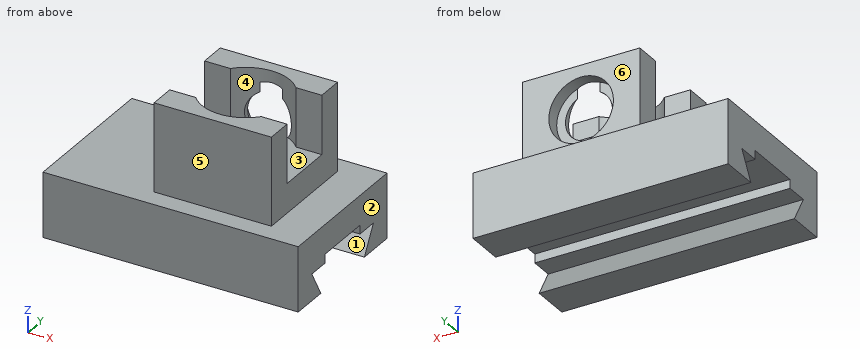
```python
from build123d import *

# Parameters (mm, degrees)
SKETCH1_W         = 87
SKETCH1_H         = 50.982
BASE_YELLOW_DEPTH = 22
SKETCH5_W         = 40
SKETCH5_H         = 38
BASE_RED_DEPTH    = 30
BASE_TURKIZ_DEPTH = 88
SKETCH2_R         = 11
COUNTERBOR_DEPTH  = 4.5
SKETCH7_R         = 15
SKETCH7_W         = 40
SKETCH7_H         = 20
BASE_PURPLE_DEPTH = 20
SKETCH2_5_R       = 8
COUNTERBOR2_DEPTH = 8


with BuildPart() as part:
    # Sketch1 → base-yellow (new body)
    with BuildSketch(Plane.XY):
        Rectangle(SKETCH1_W, SKETCH1_H)
    extrude(amount=-BASE_YELLOW_DEPTH)

    # Sketch5 → base-red (add)
    with BuildSketch(Plane.XY):
        with Locations((10.5, 0)):
            Rectangle(SKETCH5_W, SKETCH5_H)
    extrude(amount=BASE_RED_DEPTH)

    # Sketch8 → base-turkiz (cut, through all)
    with BuildSketch(Plane.ZY.offset(43.5)):
        Polygon((-10, 10), (-10, -10), (-13, -10), (-13, -17.696152423), (-22, -12.5), (-22, 12.5), (-13, 17.696152423), (-13, 10), align=None)
    extrude(amount=-BASE_TURKIZ_DEPTH, mode=Mode.SUBTRACT)

    # Sketch2 → counterbor (cut)
    with BuildSketch(Plane(origin=(0, 19, -19), x_dir=(1, 0, 0), z_dir=(0, -1, 0))):
        with Locations((10.5, 34)):
            Circle(SKETCH2_R)
    extrude(amount=COUNTERBOR_DEPTH, mode=Mode.SUBTRACT)

    # Sketch7 → base-purple (cut)
    with BuildSketch(Plane.XY.offset(30)):
        with Locations((10.5, 0)):
            Circle(SKETCH7_R)
        with Locations((10.5, 0)):
            Rectangle(SKETCH7_W, SKETCH7_H)
    extrude(amount=-BASE_PURPLE_DEPTH, mode=Mode.SUBTRACT)

    # Sketch2<5> → counterbor2 (cut)
    with BuildSketch(Plane(origin=(0, 19, -19), x_dir=(1, 0, 0), z_dir=(0, -1, 0))):
        with Locations((10.5, 34)):
            Circle(SKETCH2_5_R)
    extrude(amount=COUNTERBOR2_DEPTH, mode=Mode.SUBTRACT)


solid = part.part
```
Could you check a few things on this model? Use its own coordinates, in mm. Face numbers are marked on the shaded views. A direction names the side the tool comes from. Round coordinates to 2 decimals unless told otherwise and drop trailing zeros. Loops run counter-clockwise (first coordinate to the right, second up) from the corner with the lowest first, then second, coordinate; pieces in that order, holes last.
Q1. I want a section at A-A (x = 10.5). Write out the boundary of the cut face in (y, z), and give its area (3 significant figures).
Q2. I want a section at D-D (y = -8). Write out the boundary of the cut face in (x, z), and give its area (3 significant figures).
Q3. For P1, Ø2.5, axis at x = -4.5, z = 22.5, coming from the +Y side; P2, Ø4.5, axis at x = 26.5, z = 22, coming from the -Y side; P3, Ø6, axis at y = 10.5, z = 20.5, coming from the +X side, each with a flat end and sliding along its axis, tell me the tip position at first contact or that it passes through.
Q4. On a 3-axis mill with a long thin cutter (end or side, diameter ignored), from which of +Z, -Z, +X, -X, +Y, -Y can I reach the whole of each face in a straight line? I mean the marked faces 4, 5 and 6. Say none if no direction works.
Q5. I want a section at B-B (x = 27.5). Write out the boundary of the cut face in (y, z).
Q6. I want a section at C-C (z = 19.5). Write out the boundary of the cut face in (x, y).
Q7. Please list where these lines run through material, in increasing order: L1, parallel to X at y = 17.35, z = 15; L2, parallel to Z at x = 10.5, y = 15.55; L3, parallel to Z at x = 10.5, y = 15.7.
Q8. Thinking about a two-plate mould opening in Z: for the marked faces 1, 2 and 3, which applies, pulls with the +Z half, pulls with the -Z half, needs draft (parallel to the pull), parting line crosses it, or undercut?
Answer below:
1. outline: (-25.49, -22) - (-12.5, -22) - (-17.7, -13) - (-10, -13) - (-10, -10) - (10, -10) - (10, -13) - (17.7, -13) - (12.5, -22) - (25.49, -22) - (25.49, 0) - (19, 0) - (19, 4) - (14.5, 4) - (14.5, 7) - (11, 7) - (11, 10) - (-15, 10) - (-15, 30) - (-19, 30) - (-19, 0) - (-25.49, 0) - close; (15, 26) - (19, 26) - (19, 30) - (15, 30) - close
1. area: 1,230 mm2
2. outline: (-43.5, -10) - (43.5, -10) - (43.5, 0) - (30.5, 0) - (30.5, 10) - (-9.5, 10) - (-9.5, 0) - (-43.5, 0) - close
2. area: 1,270 mm2
3. P1: stops at y = 19
3. P2: stops at y = -19
3. P3: stops at x = 30.5
4. face 4: +Z
4. face 5: +Z, +X, -X, -Y
4. face 6: +Z, +X, -X, +Y
5. outline: (-25.49, -22) - (-12.5, -22) - (-17.7, -13) - (-10, -13) - (-10, -10) - (10, -10) - (10, -13) - (17.7, -13) - (12.5, -22) - (25.49, -22) - (25.49, 0) - (19, 0) - (19, 30) - (10, 30) - (10, 10) - (-10, 10) - (-10, 30) - (-19, 30) - (-19, 0) - (-25.49, 0) - close
6. outline: (-9.5, -19) - (30.5, -19) - (30.5, -10) - (21.68, -10) arc R15 cw to (-0.68, -10) - (-9.5, -10) - close; (-9.5, 10) - (-0.68, 10) arc R15 cw to (3.89, 13.46) - (3.89, 14.5) - (0.46, 14.5) - (0.46, 19) - (-9.5, 19) - close; (17.11, 13.46) arc R15 cw to (21.68, 10) - (30.5, 10) - (30.5, 19) - (20.54, 19) - (20.54, 14.5) - (17.11, 14.5) - close
7. L1: x = -9.5 to -0.5, 21.5 to 30.5
7. L2: z = -22 to -16.72, -13 to 4, 26 to 30
7. L3: z = -22 to -16.46, -13 to 4, 26 to 30
8. face 1: undercut
8. face 2: needs draft
8. face 3: pulls with the +Z half
